```python
from build123d import *

# Parameters (mm, degrees)
SKETCH_235_R             = 70
EXTRUDE_1_DEPTH          = 130
SKETCH_315_R             = 62.5
CUT_EXTRUDE_1_DEPTH      = 120
CUT_EXTRUDE_2_DEPTH      = 110
SKETCH_5_R               = 35
CUT_EXTRUDE_3_DEPTH      = 110
SKETCH_9_R               = 2.5
CUT_EXTRUDE_5_DEPTH      = 30
PATTERN_CIRCULAR_2_COUNT = 4


with BuildPart() as part:
    # Sketch 235 → Бобышка-Вытянуть1 (new body)
    with BuildSketch(Plane(origin=(0, 0, 0), x_dir=(1, 0, 0), z_dir=(0, 1, 0))):
        Circle(SKETCH_235_R)
    extrude(amount=EXTRUDE_1_DEPTH)

    # Sketch 315 → Вырез-Вытянуть1 (cut)
    with BuildSketch(Plane(origin=(0, 130, 0), x_dir=(1, 0, 0), z_dir=(0, 1, 0))):
        Circle(SKETCH_315_R)
    extrude(amount=-CUT_EXTRUDE_1_DEPTH, mode=Mode.SUBTRACT)

    # Sketch 408 → Вырез-Вытянуть2 (cut)
    with BuildSketch(Plane(origin=(0, 130, 0), x_dir=(1, 0, 0), z_dir=(0, 1, 0))):
        Polygon((-11.607142857, -61.412736746), (-13, -68.782265156), (0, -74.034115552), (13, -68.782265156), (11.607142857, -61.412736746), align=None)
    extrude(amount=-CUT_EXTRUDE_2_DEPTH, mode=Mode.SUBTRACT)

    # Эскиз5 → Вырез-Вытянуть3 (cut)
    with BuildSketch(Plane.XZ):
        Circle(SKETCH_5_R)
    extrude(amount=-CUT_EXTRUDE_3_DEPTH, mode=Mode.SUBTRACT)

    # Эскиз9 → Вырез-Вытянуть5 (cut)
    with BuildSketch(Plane(origin=(70, 0, 0), x_dir=(0, 0, -1), z_dir=(1, 0, 0))):
        with Locations((0, 25)):
            Circle(SKETCH_9_R)
    cut_extrude_5 = extrude(amount=-CUT_EXTRUDE_5_DEPTH, mode=Mode.SUBTRACT)

    # Круговой массив2: Вырез-Вытянуть5 ×4 about axis
    pattern_circular_2_axis = Axis((0, -1.889670697, 0), (0, 1, 0))
    for i in range(1, PATTERN_CIRCULAR_2_COUNT):
        add(cut_extrude_5.rotate(pattern_circular_2_axis, i * 360 / PATTERN_CIRCULAR_2_COUNT), mode=Mode.SUBTRACT)


solid = part.part
```
The listing builds one solid part. Answer for the finished solid, in the listing's coordinates (mm). A direction names the side the tool comes from. Give positions to 0.01 mm unless a question says otherwise; leave off trailing zeros. Order: outer loops, then holes, each group sorted by start corner. A loop starts at its lowest first (then second) coordinate and runs counter-clockwise, first axis right, second up.
1) Find section C-C on y = 25. Write down the section's boundary in (x, z).
Reported:
outline: (-69.96, -2.5) arc R70 ccw to (-2.5, -69.96) - (-2.5, -62.45) arc R62.5 cw to (-62.45, -2.5) - close; (-69.96, 2.5) - (-62.45, 2.5) arc R62.5 cw to (-11.61, 61.41) - (-13, 68.78) arc R70 ccw to start; (2.5, -69.96) arc R70 ccw to (69.96, -2.5) - (62.45, -2.5) arc R62.5 cw to (2.5, -62.45) - close; (11.61, 61.41) arc R62.5 cw to (62.45, 2.5) - (69.96, 2.5) arc R70 ccw to (13, 68.78) - close
2) For faces 1 (the face through (-12.294, 75.77, 65.046)), 2 (the face through (-62.44, 70.84, -2.75)), 3 (the face through (-28, 5, -21)), determine the directions among +Z, -Z, +X, -X, +Y, -Y from which every point of the face is accessible in a straight line to the end or side of a thin tool.
Reported:
face 1: +Z, +Y
face 2: +Y
face 3: +Y, -Y
3) Find section A-A on z = 0. Write down the section's boundary in (x, y), then the cut area to 4 significant figures.
Reported:
outline: (-70, 0) - (-35, 0) - (-35, 10) - (-62.5, 10) - (-62.5, 22.5) - (-70, 22.5) - close; (-70, 27.5) - (-62.5, 27.5) - (-62.5, 130) - (-70, 130) - close; (35, 0) - (70, 0) - (70, 22.5) - (62.5, 22.5) - (62.5, 10) - (35, 10) - close; (62.5, 27.5) - (70, 27.5) - (70, 130) - (62.5, 130) - close
area: 2,425 mm2
4) Find section D-D on x = -17.5. Write down the section's boundary in (y, z), then the cut area to 3 significant figures.
Reported:
outline: (0, -67.78) - (130, -67.78) - (130, -60) - (10, -60) - (10, -30.31) - (0, -30.31) - close; (0, 30.31) - (10, 30.31) - (10, 60) - (130, 60) - (130, 67.78) - (0, 67.78) - close
area: 2,620 mm2
5) Find section B-B on x = 0. Write down the section's boundary in (y, z), then the cut area to 3 significant figures.
Reported:
outline: (0, -70) - (22.5, -70) - (22.5, -62.5) - (10, -62.5) - (10, -35) - (0, -35) - close; (0, 35) - (10, 35) - (10, 62.5) - (20, 62.5) - (20, 70) - (0, 70) - close; (27.5, -70) - (130, -70) - (130, -62.5) - (27.5, -62.5) - close
area: 1,640 mm2
6) Consider line 1 along Y through (x, z) = (0, -66); line 2 along X through (y, z) = (119, 0.5); line 3 along Z through (x, y) = (0, 7). Determine where each line is inside the solid, lowest interval first.
Reported:
line 1: y = 0 to 22.5, 27.5 to 130
line 2: x = -70 to -62.5, 62.5 to 70
line 3: z = -70 to -35, 35 to 70
7) Given P1, Ø6, axis at x = -21.5, y = 110.5, coming from the -Z side; P2, Ø1.5, axis at x = -41.5, z = 6, coming from the +Y side; P3, Ø3, axis at x = 0, y = 25, coming from the -Z side; P4, Ø7, axis at x = 0, z = 65, coming from the +Y side, each flat-ended and moving along its own axis, determine where each tip first touches the part or whether it passes through.
Reported:
P1: stops at z = -67.51
P2: stops at y = 10
P3: passes through
P4: stops at y = 20
8) Determine the mould class of faces 4 (the face through (-55.55, 64.09, 42.594)), 5 (the face through (-32, 0, 15)), 6 (the face through (27, 10, 27)) for opening direction X: pulls with the +X half, pulls with the -X half, needs draft (parallel to the pull), parting line crosses it, or undercut.
Reported:
face 4: parting line crosses it
face 5: needs draft
face 6: undercut
